Read the model definition and answer for the solid it produces. Units are mm, in the model's axes. Face numbers are marked on the shaded views. A direction names the side the tool comes from. Coordinates: 2 decimals unless noted, no trailing zeros. Order: outer loops, then holes, each group sorted by start corner. A loop starts at its lowest first (then second) coordinate and runs counter-clockwise, first axis right, second up. Notation, with made-up numbers: M 64,2.5 L 99,2.5 A25 cw 99,38.5 Z; hole C 6.5,78.25 d4. An arc over 180 degrees is marked long. Write each question's results on one line, items separated by ' | '.
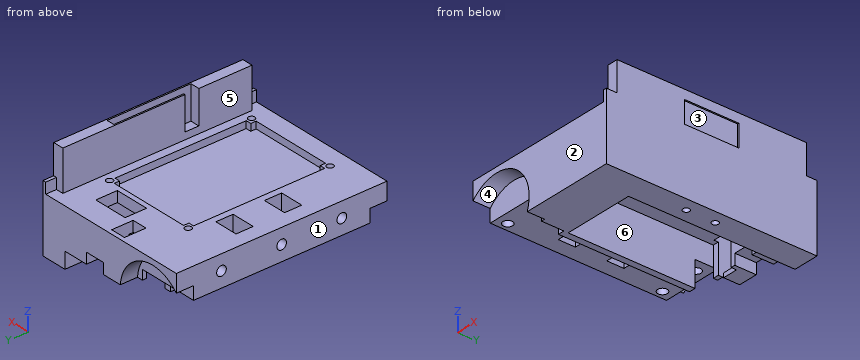
```python
from build123d import *

# Parameters (mm, degrees)
SKETCH1_W           = 72
SKETCH1_H           = 26.25
BOSS_EXTRUDE1_DEPTH = 98
SKETCH3_W           = 24
SKETCH3_H           = 12
CUT_EXTRUDE2_DEPTH  = 98
SKETCH4_W           = 1
SKETCH4_H           = 14.25
BOSS_EXTRUDE2_DEPTH = 98
SKETCH8_R           = 17.75
CUT_EXTRUDE6_DEPTH  = 8
CUT_EXTRUDE7_START  = -8
SKETCH9_R           = 17.75
CUT_EXTRUDE7_DEPTH  = 8
SKETCH10_R          = 2.25
CUT_EXTRUDE8_DEPTH  = 4.25
SKETCH11_W          = 33
SKETCH11_H          = 67.5
CUT_EXTRUDE9_DEPTH  = 21.25
SKETCH12_W          = 33
SKETCH12_H          = 7.5
CUT_EXTRUDE10_DEPTH = 21.25
SKETCH13_W          = 9.5
SKETCH13_H          = 10
CUT_EXTRUDE11_DEPTH = 21.25
SKETCH14_W          = 5
SKETCH14_H          = 5
CUT_EXTRUDE13_DEPTH = 101.25
SKETCH17_W          = 7
SKETCH17_H          = 8
CUT_EXTRUDE14_DEPTH = 7
SKETCH18_W          = 5.398243629
SKETCH18_H          = 5.439982626
BOSS_EXTRUDE3_DEPTH = 2
SKETCH19_W          = 16
SKETCH19_H          = 10
CUT_EXTRUDE15_DEPTH = 12
SKETCH22_R          = 1.5
CUT_EXTRUDE16_DEPTH = 8.2
SKETCH23_W          = 11
SKETCH23_H          = 8
CUT_EXTRUDE18_DEPTH = 125.988249448
SKETCH25_R          = 2.25
CUT_EXTRUDE20_DEPTH = 10.25
SKETCH26_W          = 7
SKETCH26_H          = 8
CUT_EXTRUDE21_DEPTH = 124.057913195
SKETCH28_W          = 7.2
SKETCH28_H          = 8.135980894
BOSS_EXTRUDE6_DEPTH = 2
SKETCH31_R          = 1.5
CUT_EXTRUDE24_DEPTH = 3.25
SKETCH32_W          = 5
SKETCH32_H          = 98
BOSS_EXTRUDE7_DEPTH = 18.75
SKETCH34_W          = 5
SKETCH34_H          = 5
CUT_EXTRUDE27_DEPTH = 13.75
SKETCH35_W          = 3.5
SKETCH35_H          = 5
CUT_EXTRUDE28_DEPTH = 5
SKETCH37_W          = 10.25
SKETCH37_H          = 25.25
CUT_EXTRUDE29_DEPTH = 3
SKETCH36_W          = 3.65
SKETCH36_H          = 39
CUT_EXTRUDE30_DEPTH = 15.5
CUT_EXTRUDE31_DEPTH = 15.5
CUT_EXTRUDE32_DEPTH = 3.25
SKETCH41_W          = 7
SKETCH41_H          = 2.5
CUT_EXTRUDE33_DEPTH = 3
SKETCH42_W          = 7
SKETCH42_H          = 2
CUT_EXTRUDE34_DEPTH = 6
SKETCH43_W          = 3
SKETCH43_H          = 10.5
CUT_EXTRUDE35_DEPTH = 12


with BuildPart() as part:
    # Sketch1 → Boss-Extrude1 (new body)
    with BuildSketch(Plane(origin=(0, 0, 0), x_dir=(1, 0, 0), z_dir=(0, 1, 0))):
        with Locations((-36, -13.125)):
            Rectangle(SKETCH1_W, SKETCH1_H)
    extrude(amount=BOSS_EXTRUDE1_DEPTH)

    # Sketch3 → Cut-Extrude2 (cut)
    with BuildSketch(Plane.XZ):
        with Locations((-60, 6)):
            Rectangle(SKETCH3_W, SKETCH3_H)
    extrude(amount=-CUT_EXTRUDE2_DEPTH, mode=Mode.SUBTRACT)

    # Sketch4 → Boss-Extrude2 (add)
    with BuildSketch(Plane(origin=(0, 0, 0), x_dir=(-1, 0, 0), z_dir=(0, -1, 0))):
        with Locations((72.5, -19.125)):
            Rectangle(SKETCH4_W, SKETCH4_H)
    extrude(amount=-BOSS_EXTRUDE2_DEPTH)

    # Sketch8 → Cut-Extrude6 (cut)
    with BuildSketch(Plane.XZ):
        with Locations((-60, 6)):
            Circle(SKETCH8_R)
    extrude(amount=-CUT_EXTRUDE6_DEPTH, mode=Mode.SUBTRACT)

    # Sketch9 → Cut-Extrude7 (cut)
    with BuildSketch(Plane(origin=(0, 98, 0), x_dir=(1, 0, 0), z_dir=(0, 1, 0)).offset(CUT_EXTRUDE7_START)):
        with Locations((-60, -6)):
            Circle(SKETCH9_R)
    extrude(amount=CUT_EXTRUDE7_DEPTH, mode=Mode.SUBTRACT)

    # Sketch10 → Cut-Extrude8 (cut)
    with BuildSketch(Plane(origin=(0, 0, 12), x_dir=(-1, 0, 0), z_dir=(0, 0, -1))):
        with Locations((69.25, 85)):
            Circle(SKETCH10_R)
        with Locations((50.75, 85)):
            Circle(SKETCH10_R)
        with Locations((69.25, 13)):
            Circle(SKETCH10_R)
        with Locations((50.75, 13)):
            Circle(SKETCH10_R)
    extrude(amount=-CUT_EXTRUDE8_DEPTH, mode=Mode.SUBTRACT)

    # Sketch11 → Cut-Extrude9 (cut)
    with BuildSketch(Plane(origin=(0, 0, 0), x_dir=(-1, 0, 0), z_dir=(0, 0, -1))):
        with Locations((28.5, 54.25)):
            Rectangle(SKETCH11_W, SKETCH11_H)
    extrude(amount=-CUT_EXTRUDE9_DEPTH, mode=Mode.SUBTRACT)

    # Sketch12 → Cut-Extrude10 (cut)
    with BuildSketch(Plane(origin=(0, 98, 0), x_dir=(1, 0, 0), z_dir=(0, 1, 0))):
        with Locations((-28.5, -3.75)):
            Rectangle(SKETCH12_W, SKETCH12_H)
    extrude(amount=-CUT_EXTRUDE10_DEPTH, mode=Mode.SUBTRACT)

    # Sketch13 → Cut-Extrude11 (cut)
    with BuildSketch(Plane(origin=(0, 98, 0), x_dir=(1, 0, 0), z_dir=(0, 1, 0))):
        with Locations((-28.5, -7.5)):
            Rectangle(SKETCH13_W, SKETCH13_H)
    extrude(amount=-CUT_EXTRUDE11_DEPTH, mode=Mode.SUBTRACT)

    # Sketch14 → Cut-Extrude13 (cut)
    with BuildSketch(Plane(origin=(0, 20.5, 0), x_dir=(1, 0, 0), z_dir=(0, 1, 0))):
        with Locations((-39.5, -12)):
            Rectangle(SKETCH14_W, SKETCH14_H)
    extrude(amount=CUT_EXTRUDE13_DEPTH, mode=Mode.SUBTRACT)

    # Sketch17 → Cut-Extrude14 (cut)
    with BuildSketch(Plane(origin=(0, 0, 7.5), x_dir=(-1, 0, 0), z_dir=(0, 0, -1))):
        with Locations((38.75, 92)):
            Rectangle(SKETCH17_W, SKETCH17_H)
    extrude(amount=-CUT_EXTRUDE14_DEPTH, mode=Mode.SUBTRACT)

    # Sketch18 → Boss-Extrude3 (add)
    with BuildSketch(Plane(origin=(0, 98, 0), x_dir=(1, 0, 0), z_dir=(0, 1, 0))):
        with Locations((-39.480706385, -11.994977786)):
            Rectangle(SKETCH18_W, SKETCH18_H)
    extrude(amount=-BOSS_EXTRUDE3_DEPTH)

    # Sketch19 → Cut-Extrude15 (cut)
    with BuildSketch(Plane.XY.offset(26.25)):
        with Locations((-24, 82)):
            Rectangle(SKETCH19_W, SKETCH19_H)
    extrude(amount=-CUT_EXTRUDE15_DEPTH, mode=Mode.SUBTRACT)

    # Sketch22 → Cut-Extrude16 (cut)
    with BuildSketch(Plane(origin=(0, 0, 0), x_dir=(-1, 0, 0), z_dir=(0, 0, -1))):
        with Locations((6, 55.73)):
            Circle(SKETCH22_R)
        with Locations((6, 42.27)):
            Circle(SKETCH22_R)
    extrude(amount=-CUT_EXTRUDE16_DEPTH, mode=Mode.SUBTRACT)

    # Sketch23 → Cut-Extrude18 (cut, through all)
    with BuildSketch(Plane.XY.offset(26.25)):
        with Locations((-60.5, 37.7)):
            Rectangle(SKETCH23_W, SKETCH23_H)
        with Locations((-60.5, 60.3)):
            Rectangle(SKETCH23_W, SKETCH23_H)
    extrude(amount=-CUT_EXTRUDE18_DEPTH, mode=Mode.SUBTRACT)

    # Sketch25 → Cut-Extrude20 (cut)
    with BuildSketch(Plane.ZY.offset(73)):
        with Locations((19.125, 77)):
            Circle(SKETCH25_R)
        with Locations((19.125, 49)):
            Circle(SKETCH25_R)
        with Locations((19.125, 21)):
            Circle(SKETCH25_R)
    extrude(amount=-CUT_EXTRUDE20_DEPTH, mode=Mode.SUBTRACT)

    # Sketch26 → Cut-Extrude21 (cut, through all)
    with BuildSketch(Plane(origin=(0, 0, 14.5), x_dir=(-1, 0, 0), z_dir=(0, 0, -1))):
        with Locations((38.75, 92)):
            Rectangle(SKETCH26_W, SKETCH26_H)
    extrude(amount=-CUT_EXTRUDE21_DEPTH, mode=Mode.SUBTRACT)

    # Sketch28 → Boss-Extrude6 (add)
    with BuildSketch(Plane(origin=(0, 0, 7.5), x_dir=(-1, 0, 0), z_dir=(0, 0, -1))):
        with Locations((38.666345703, 92.067990447)):
            Rectangle(SKETCH28_W, SKETCH28_H)
    extrude(amount=-BOSS_EXTRUDE6_DEPTH)

    # Sketch31 → Cut-Extrude24 (cut)
    with BuildSketch(Plane.XY.offset(26.25)):
        with Locations((-52.007752906, 74.651528785)):
            Circle(SKETCH31_R)
        with Locations((-9.007752906, 74.651528785)):
            Circle(SKETCH31_R)
        with Locations((-9.007752906, 8.625682812)):
            Circle(SKETCH31_R)
        with Locations((-52.007752906, 8.625682812)):
            Circle(SKETCH31_R)
    extrude(amount=-CUT_EXTRUDE24_DEPTH, mode=Mode.SUBTRACT)

    # Sketch32 → Boss-Extrude7 (add)
    with BuildSketch(Plane.XY.offset(26.25)):
        with Locations((-2.5, 49)):
            Rectangle(SKETCH32_W, SKETCH32_H)
    extrude(amount=BOSS_EXTRUDE7_DEPTH)

    # Sketch34 → Cut-Extrude27 (cut)
    with BuildSketch(Plane.XY.offset(45)):
        with Locations((-2.5, 95.5)):
            Rectangle(SKETCH34_W, SKETCH34_H)
        with Locations((-2.5, 2.5)):
            Rectangle(SKETCH34_W, SKETCH34_H)
    extrude(amount=-CUT_EXTRUDE27_DEPTH, mode=Mode.SUBTRACT)

    # Sketch35 → Cut-Extrude28 (cut)
    with BuildSketch(Plane.XY.offset(31.25)):
        with Locations((-3.25, 95.5)):
            Rectangle(SKETCH35_W, SKETCH35_H)
        with Locations((-3.25, 2.5)):
            Rectangle(SKETCH35_W, SKETCH35_H)
    extrude(amount=-CUT_EXTRUDE28_DEPTH, mode=Mode.SUBTRACT)

    # Sketch37 → Cut-Extrude29 (cut)
    with BuildSketch(Plane(origin=(0, 0, 0), x_dir=(0, 0, -1), z_dir=(1, 0, 0))):
        with Locations((-35.625, 49)):
            Rectangle(SKETCH37_W, SKETCH37_H)
    extrude(amount=-CUT_EXTRUDE29_DEPTH, mode=Mode.SUBTRACT)

    # Sketch36 → Cut-Extrude30 (cut)
    with BuildSketch(Plane.XY.offset(45)):
        with Locations((-2.5, 49.25)):
            Rectangle(SKETCH36_W, SKETCH36_H)
    extrude(amount=-CUT_EXTRUDE30_DEPTH, mode=Mode.SUBTRACT)

    # Sketch38 → Cut-Extrude31 (cut)
    with BuildSketch(Plane.XY.offset(45)):
        Polygon((-4.325, 30.125), (-4.325, 29.75), (-5, 29.75), (-5.005, 30.125), (-5.005, 36.125), (-4.325, 36.125), align=None)
    extrude(amount=-CUT_EXTRUDE31_DEPTH, mode=Mode.SUBTRACT)

    # Sketch39 → Cut-Extrude32 (cut)
    with BuildSketch(Plane.XY.offset(26.25)):
        Polygon((-49.507752906, 72.151528785), (-52.007752906, 72.151528785), (-52.007752906, 11.125682812), (-49.507752906, 11.125682812), (-49.507752906, 8.625682812), (-11.507752906, 8.625682812), (-11.507752906, 11.125682812), (-9.007752906, 11.125682812), (-9.007752906, 72.151528785), (-11.507752906, 72.151528785), (-11.507752906, 74.651528785), (-49.507752906, 74.651528785), align=None)
    extrude(amount=-CUT_EXTRUDE32_DEPTH, mode=Mode.SUBTRACT)

    # Sketch41 → Cut-Extrude33 (cut)
    with BuildSketch(Plane(origin=(0, 0, 7.5), x_dir=(-1, 0, 0), z_dir=(0, 0, -1))):
        with Locations((38.75, 89.25)):
            Rectangle(SKETCH41_W, SKETCH41_H)
    extrude(amount=-CUT_EXTRUDE33_DEPTH, mode=Mode.SUBTRACT)

    # Sketch42 → Cut-Extrude34 (cut)
    with BuildSketch(Plane.XY.offset(26.25)):
        with Locations((-38.75, 87)):
            Rectangle(SKETCH42_W, SKETCH42_H)
    extrude(amount=-CUT_EXTRUDE34_DEPTH, mode=Mode.SUBTRACT)

    # Sketch43 → Cut-Extrude35 (cut)
    with BuildSketch(Plane(origin=(0, 0, 0), x_dir=(-1, 0, 0), z_dir=(0, 0, -1))):
        with Locations((46.5, 84.75)):
            Rectangle(SKETCH43_W, SKETCH43_H)
        with Locations((46.5, 13.25)):
            Rectangle(SKETCH43_W, SKETCH43_H)
    extrude(amount=-CUT_EXTRUDE35_DEPTH, mode=Mode.SUBTRACT)


solid = part.part
```
(1) The part is cut by section A-A, the plane z = 39.5. Write down the section's boundary in (x, y) (3 decimals), then the cut area to 3 significant figures.
Conclusion:
outline: M -5,5 L 0,5 L 0,36.375 L -0.675,36.375 L -0.675,29.75 L -5,29.75 Z; M -5,36.125 L -4.325,36.125 L -4.325,68.75 L -0.675,68.75 L -0.675,61.625 L 0,61.625 L 0,93 L -5,93 Z | area: 276 mm²
(2) The part is cut by section C-C, the plane x = -39.5. Write down the section's boundary in (y, z).
Conclusion:
outline: M 0,0 L 20.5,0 L 20.5,21.25 L 86,21.25 L 86,26.25 L 74.65,26.25 L 74.65,23 L 8.63,23 L 8.63,26.25 L 0,26.25 Z; M 90.5,7.5 L 98,7.5 L 98,26.25 L 96,26.25 L 96,9.5 L 90.5,9.5 Z
(3) Given pin 1 (12 mm diameter, centred on y = 69.5, z = 37.5, fed in from +X); pin 2 (2.5 mm diameter, centred on x = -69.25, y = 13, fed in from +Z); pin 3 (5 mm diameter, centred on x = -51.5, y = 13, fed in from -Z); pin 4 (1.3 mm diameter, centred on x = -2, y = 55, fed in from +Z), each flat-ended and moving along its own axis, determine where each tip first touches the part or whether it passes through.
Conclusion:
pin 1: x = 0 | pin 2: z = 26.25 | pin 3: z = 12 | pin 4: z = 29.5
(4) Straight lines are drawn through the part: line 1 (Y direction, x = -6, z = 2); line 2 (Y direction, x = -50.75, z = 15.3); line 3 (Y direction, x = -64.5, z = 19). For each, find the intervals that lie inside material, in ascending order.
Conclusion:
line 1: 0 to 40.77, 43.77 to 54.23, 57.23 to 98 | line 2: 8 to 10.75, 15.25 to 82.75, 87.25 to 90 | line 3: 8 to 18.75, 23.25 to 33.7, 41.7 to 46.75, 51.25 to 56.3, 64.3 to 74.75, 79.25 to 90
(5) For the marked faces 4, 5 and 6, determine the directions among +Z, -Z, +X, -X, +Y, -Y from which every point of the face is accessible in a straight line to the end or side of a thin tool.
Conclusion:
face 4: -Y | face 5: +Z, -X, +Y, -Y | face 6: -Z
(6) The part is cut by section B-B, the plane y = 49. Write down the section's boundary in (x, z) (3 decimals), then the cut area to 3 significant figures.
Conclusion:
outline: M -73,12 L -48,12 L -48,0 L -45,0 L -45,21.25 L -12,21.25 L -12,0 L 0,0 L 0,30.5 L -0.675,30.5 L -0.675,29.5 L -4.325,29.5 L -4.325,45 L -5,45 L -5,26.25 L -9.008,26.25 L -9.008,23 L -52.008,23 L -52.008,26.25 L -73,26.25 L -73,21.375 L -62.75,21.375 L -62.75,16.875 L -73,16.875 Z; M -0.675,40.75 L 0,40.75 L 0,45 L -0.675,45 Z | area: 759 mm²
(7) The part is cut by section D-D, the plane x = -69.25. Write down the section's boundary in (y, z) (3 decimals).
Conclusion:
outline: M 0,21.149 L 8,21.149 L 8,12 L 10.75,12 L 10.75,16.25 L 15.25,16.25 L 15.25,12 L 82.75,12 L 82.75,16.25 L 87.25,16.25 L 87.25,12 L 90,12 L 90,21.149 L 98,21.149 L 98,26.25 L 0,26.25 Z; hole C 21,19.125 d4.5; hole C 49,19.125 d4.5; hole C 77,19.125 d4.5
(8) The mould has two halves that part along X. Classify the marked faces 1, 2 and 3: pulls with the +X half, pulls with the -X half, needs draft (parallel to the pull), parting line crosses it, or undercut.
Conclusion:
face 1: pulls with the -X half | face 2: needs draft | face 3: undercut
